```python
from build123d import *

# Parameters (mm, degrees)
F1_DEPTH = 0.78
F2_R     = 0.5
F4_DEPTH = 25
F5_R     = 0.5


with BuildPart() as f1:
    # F0 (on Front) → F1 (new body)
    with BuildSketch(Plane.XZ):
        Polygon((4.6385581188, 7.5), (-6.05, 7.5), (-6.05, -7.5), (6.05, -7.5), (6.05, 6.0885581188), align=None)
    extrude(amount=F1_DEPTH)

    # F2
    f2_edges = [f1.edges().sort_by_distance(p)[0] for p in [
        (-6.05, -0.39, 7.5),
        (-6.05, -0.39, -7.5),
        (6.05, -0.39, -7.5),
        (4.638558, -0.39, 7.5),
        (6.05, -0.39, 6.088558),
    ]]
    fillet(f2_edges, radius=F2_R)

    # F3 (on face) → F4 (cut)
    with BuildSketch(Plane.XZ.offset(0.78)):
        Polygon((2.5064539127, 5.8), (-5.25, 5.8), (-5.25, -6.4), (3.55, -6.4), (3.55, 4.7564539127), align=None)
    extrude(amount=-F4_DEPTH, mode=Mode.SUBTRACT)

    # F5
    f5_edges = [f1.edges().sort_by_distance(p)[0] for p in [
        (-5.25, -0.39, 5.8),
        (-5.25, -0.39, -6.4),
        (3.55, -0.39, -6.4),
        (3.55, -0.39, 4.756454),
        (2.506454, -0.39, 5.8),
    ]]
    fillet(f5_edges, radius=F5_R)


solid = f1.part
```
For this review, take the finished solid that the model builds, in its own axes (mm). Coordinates: 2 decimals unless noted, no trailing zeros. Loops run counter-clockwise (first coordinate to the right, second up) from the corner with the lowest first, then second, coordinate; pieces in that order, holes last. Notation, with made-up numbers: (43.25, 29.25) - (91.25, 29.25) arc R34 ccw to (91.25, 68.25) - close; hole circle Ø5 at (-14, 17.25). An arc over 180 degrees is marked (long way). Use one line per item in the form item = value. Start each with the question number.
1) Take a section at C-C (z = 1.75). State the section outline as (x, y) points.
2) Take a section at B-B (y = -0.65). State the section outline as (x, z) points (3 decimals), plus the area to 3 significant figures.
3) To check wall thickness, follow probe 1 along Z at (x, y) = (2.25, -0.1); probe 2 along X at (y, z) = (-0.65, -4.5); probe 3 along X at (y, z) = (-0.25, 5). State the ranges of each line that lie inside material, in increasing order. Write a range as from..to.
4) Take a section at A-A (x = -0.5). State the section outline as (y, z) points.
5) Take a section at D-D (x = 5). State the section outline as (y, z) points.
From the geometry:
q1.outline = (-6.05, -0.78) - (-5.25, -0.78) - (-5.25, 0) - (-6.05, 0) - close; (3.55, -0.78) - (6.05, -0.78) - (6.05, 0) - (3.55, 0) - close
q2.outline = (-6.05, -7) arc R0.5 ccw to (-5.55, -7.5) - (5.55, -7.5) arc R0.5 ccw to (6.05, -7) - (6.05, 5.881) arc R0.5 ccw to (5.904, 6.235) - (4.785, 7.354) arc R0.5 ccw to (4.431, 7.5) - (-5.55, 7.5) arc R0.5 ccw to (-6.05, 7) - close; hole (-5.25, -5.9) arc R0.5 ccw to (-4.75, -6.4) - (3.05, -6.4) arc R0.5 ccw to (3.55, -5.9) - (3.55, 4.549) arc R0.5 ccw to (3.404, 4.903) - (2.653, 5.654) arc R0.5 ccw to (2.299, 5.8) - (-4.75, 5.8) arc R0.5 ccw to (-5.25, 5.3) - close
q2.area = 73.7 mm2
q3.probe_1 = -7.5..-6.4, 5.8..7.5
q3.probe_2 = -6.05..-5.25, 3.55..6.05
q3.probe_3 = -6.05..-5.25, 3.31..6.05
q4.outline = (-0.78, -7.5) - (0, -7.5) - (0, -6.4) - (-0.78, -6.4) - close; (-0.78, 5.8) - (0, 5.8) - (0, 7.5) - (-0.78, 7.5) - close
q5.outline = (-0.78, -7.5) - (0, -7.5) - (0, 7.14) - (-0.78, 7.14) - close
